Could you check a few things on this drawing? It's one solid part, dimensions in mm from its lowest x, y, z. Give positions to 0.01 mm unless a question says otherwise; leave off trailing zeros. Write each loop counter-clockwise with the first axis right and the second up, starting at its lowest first coordinate (ties: lowest second). Pieces come first, ordered by that corner, then holes.
1. Thinking about a two-plate mould opening in X: for the marked faces 1, 2 and 3, which applies, pulls with the +X half, pulls with the -X half, needs draft (parallel to the pull), parting line crosses it, or undercut?
2. I'm going to push flat-ended pins straight in: pin 1 (3 mm diameter, centred on x = 40.5, y = 12, fed in from +Z); pin 2 (1 mm diameter, centred on x = 9.5, y = 11, fed in from +Z) (1 decimal); pin 3 (1.5 mm diameter, centred on x = 20, y = 12, fed in from -Z); pin 4 (19 mm diameter, centred on x = 30, z = 30, fed in from -Y). Where does each tip first touch, or does it pass through?
3. Suppose I cut it at A-A (x = 30). Please give me the cut outline in (y, z).
4. Suppose I cut it at B-B (z = 30). Please give me the cut outline in (x, y).
5. Suppose I cut it at C-C (y = 3). Please give me the cut outline in (x, z), and give its area (3 significant figures).
6. Suppose I cut it at D-D (y = 11). Please give me the cut outline in (x, z) (1 decimal).
7. If I drill on probe 1 along X at (y, z) = (10.5, 36.5) (1 decimal); probe 2 along Z at (x, y) = (29, 8.5); probe 3 along X at (y, z) = (9, 24) (1 decimal), over which ranges is the centre line in solid material (lowest first)?
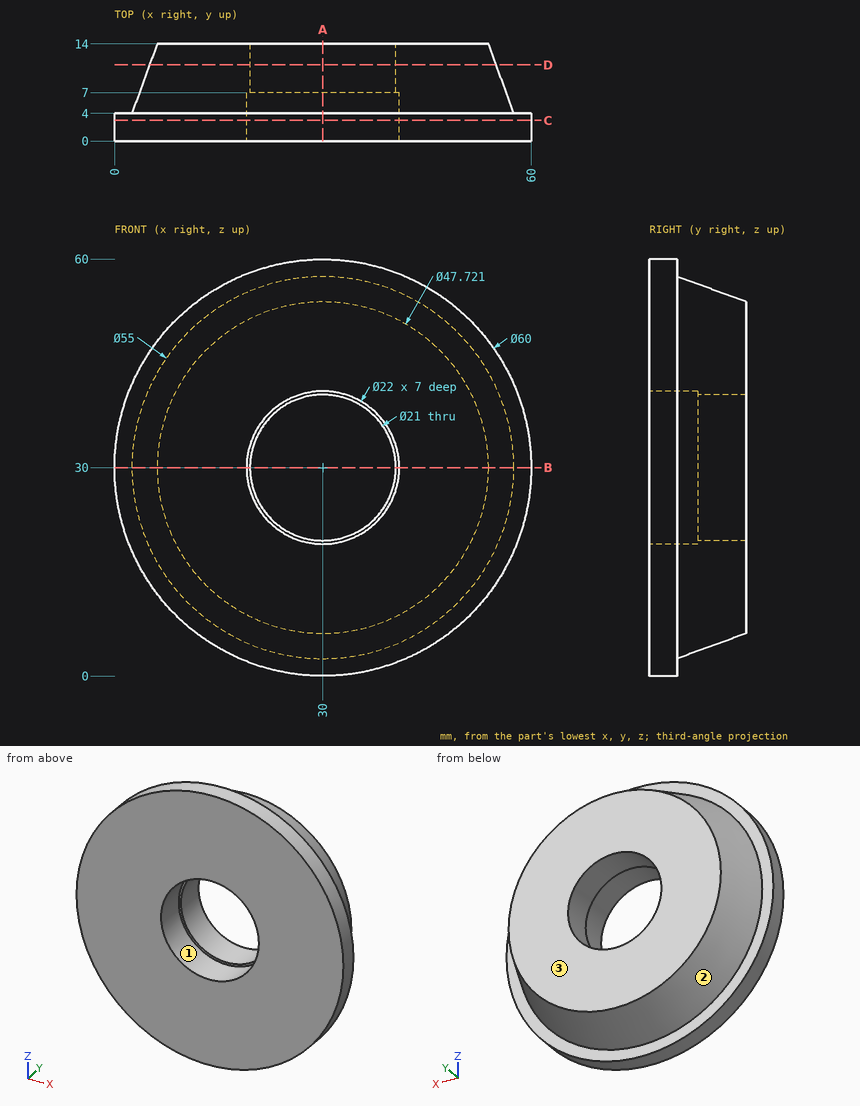
Checks:
1. face 1: undercut
1. face 2: parting line crosses it
1. face 3: needs draft
2. pin 1: stops at z = 53.12
2. pin 2: stops at z = 45
2. pin 3: stops at z = 7.1
2. pin 4: passes through
3. outline: (0, 0) - (4, 0) - (4, 2.5) - (14, 6.14) - (14, 19.5) - (7, 19.5) - (7, 19) - (0, 19) - close; (0, 41) - (7, 41) - (7, 40.5) - (14, 40.5) - (14, 53.86) - (4, 57.5) - (4, 60) - (0, 60) - close
4. outline: (0, 0) - (19, 0) - (19, 7) - (19.5, 7) - (19.5, 14) - (6.14, 14) - (2.5, 4) - (0, 4) - close; (40.5, 7) - (41, 7) - (41, 0) - (60, 0) - (60, 4) - (57.5, 4) - (53.86, 14) - (40.5, 14) - close
5. outline: circle Ø60 at (30, 30); hole circle Ø22 at (30, 30)
5. area: 2,450 mm2
6. outline: circle Ø49.9 at (30, 30); hole circle Ø21 at (30, 30)
7. probe 1: x = 5.7 to 21.8, 38.2 to 54.3
7. probe 2: z = 4.16 to 19.55, 40.45 to 55.84
7. probe 3: x = 5 to 21.4, 38.6 to 55
